from build123d import *

# Parameters (mm, degrees)
F0_W     = 127
F0_H     = 50.8
F1_DEPTH = 38.1
F2_W     = 50.8
F2_H     = 38.1
F3_DEPTH = 12.7
F4_W     = 25.4
F4_H     = 38.1
F5_DEPTH = 38.1
F6_W     = 25.4
F6_H     = 38.1
F7_DEPTH = 38.1
F8_W     = 25.4
F8_H     = 38.1
F9_DEPTH = 25.4


with BuildPart() as f1:
    # F0 (on Front) → F1 (new body)
    with BuildSketch(Plane.XZ):
        Rectangle(F0_W, F0_H)
    extrude(amount=F1_DEPTH)

    # F2 (on face) → F3 (cut)
    with BuildSketch(Plane(origin=(0, 0, -25.4), x_dir=(1, 0, 0), z_dir=(0, 0, -1))):
        with Locations((0, 19.05)):
            Rectangle(F2_W, F2_H)
    extrude(amount=-F3_DEPTH, mode=Mode.SUBTRACT)

    # F4 (on face) → F5 (cut)
    with BuildSketch(Plane.XZ.offset(38.1)):
        with Locations((-50.8, 6.35)):
            Rectangle(F4_W, F4_H)
    extrude(amount=-F5_DEPTH, mode=Mode.SUBTRACT)

    # F6 (on face) → F7 (cut)
    with BuildSketch(Plane.XZ.offset(38.1)):
        with Locations((50.8, 6.35)):
            Rectangle(F6_W, F6_H)
    extrude(amount=-F7_DEPTH, mode=Mode.SUBTRACT)

    # F8 (on face) → F9 (cut)
    with BuildSketch(Plane.XY.offset(25.4)):
        with Locations((0, -19.05)):
            Rectangle(F8_W, F8_H)
    extrude(amount=-F9_DEPTH, mode=Mode.SUBTRACT)


solid = f1.part
Build history of the part. All positions in model axes, mm. A direction names the side the tool comes from. Round coordinates to 2 decimals unless told otherwise and drop trailing zeros. Write each loop counter-clockwise with the first axis right and the second up, starting at its lowest first coordinate (ties: lowest second). Pieces come first, ordered by that corner, then holes. Notation, with made-up numbers: (-19.5, 73) -> (22.5, 73) arc R4 cw to (22.5, 77) -> close; hole circle Ø2 at (62.25, -31.5). An arc over 180 degrees is marked (long way). Write item = value, one per line.
(1) Flat gauge pins, fed straight in: pin 1 (12.5 mm diameter, centred on x = -54, y = -23, fed in from +Z); pin 2 (20.5 mm diameter, centred on y = -14, z = 8, fed in from -X); pin 3 (3 mm diameter, centred on x = 8.5, y = -12.5, fed in from -Z). Where does each tip first touch, or does it go through?
Answer:
pin_1 = -12.7
pin_2 = -38.1
pin_3 = -12.7
(2) Band-saw the part on D-D (x = -18.5). Give the cut face in (y, z), then the cut area to 3 significant figures.
Answer:
outline = (-38.1, -12.7) -> (0, -12.7) -> (0, 25.4) -> (-38.1, 25.4) -> close
area = 1,450 mm2
(3) Band-saw the part on B-B (y = -20.5). Give the cut face in (x, z), then the cut area to 3 significant figures.
Answer:
outline = (-63.5, -25.4) -> (-25.4, -25.4) -> (-25.4, -12.7) -> (25.4, -12.7) -> (25.4, -25.4) -> (63.5, -25.4) -> (63.5, -12.7) -> (38.1, -12.7) -> (38.1, 25.4) -> (12.7, 25.4) -> (12.7, 0) -> (-12.7, 0) -> (-12.7, 25.4) -> (-38.1, 25.4) -> (-38.1, -12.7) -> (-63.5, -12.7) -> close
area = 3,230 mm2
(4) Band-saw the part on A-A (z = 16). Give the cut face in (x, y).
Answer:
outline = (-38.1, -38.1) -> (-12.7, -38.1) -> (-12.7, 0) -> (-38.1, 0) -> close; (12.7, -38.1) -> (38.1, -38.1) -> (38.1, 0) -> (12.7, 0) -> close
(5) Tool access for faces 1 (the face through (12.7, -19, 13)), 2 (the face through (-25.4, -19, -19)), 3 (the face through (51, -19, -12.7)), 4 (the face through (-38.1, -19, 6)): list every direction of +Z, -Z, +X, -X, +Y, -Y with a clear straight run to the whole face (end or side of a thin tool).
Answer:
face_1 = +Z, +Y, -Y
face_2 = -Z, +Y, -Y
face_3 = +Z, +X, +Y, -Y
face_4 = +Z, -X, +Y, -Y
(6) Band-saw the part on C-C (z = -22). Give the cut face in (x, y), then the cut area to 3 significant figures.
Answer:
outline = (-63.5, -38.1) -> (-25.4, -38.1) -> (-25.4, 0) -> (-63.5, 0) -> close; (25.4, -38.1) -> (63.5, -38.1) -> (63.5, 0) -> (25.4, 0) -> close
area = 2,900 mm2
(7) Probe L1, parallel to X at y = -14, z = 6.5; L2, parallel to X at y = -30, z = -19; L3, parallel to Z at x = -58, y = -29. List the from-to ranges inside material, lowest first.
Answer:
L1 = -38.1 to -12.7, 12.7 to 38.1
L2 = -63.5 to -25.4, 25.4 to 63.5
L3 = -25.4 to -12.7
